```python
from build123d import *

# Parameters (mm, degrees)
CYLINDER005_R     = 2.2
CYLINDER005_DEPTH = 32
ARRAY004_X_COUNT  = 2
ARRAY004_X_PITCH  = 40
ARRAY004_Y_COUNT  = 2
ARRAY004_Y_PITCH  = 90
BOX005_W          = 62
BOX005_H          = 108
BOX005_DEPTH      = 32


with BuildPart() as psu_mockup_hole_array:
    # Cylinder005 → Cylinder005 (new body)
    with BuildSketch(Plane.XY):
        Circle(CYLINDER005_R)
    extrude(amount=CYLINDER005_DEPTH)

    # Array004 X: psu mockup hole array ×2


with BuildPart() as psu_mockup_hole_array_1:
    add(psu_mockup_hole_array.part)
    with Locations(*[(i * ARRAY004_X_PITCH, 0, 0) for i in range(1, ARRAY004_X_COUNT)]):
        add(psu_mockup_hole_array.part)

    # Array004 Y: psu mockup hole array ×2


with BuildPart() as psu_mockup_hole_array_2:
    add(psu_mockup_hole_array_1.part)
    with Locations(*[(0, i * ARRAY004_Y_PITCH, 0) for i in range(1, ARRAY004_Y_COUNT)]):
        add(psu_mockup_hole_array_1.part)


with BuildPart() as psu_mockup_hole_array_3:
    # Array004 placement: moved
    add(psu_mockup_hole_array_2.part.moved(Location((11, 9, 0))))


with BuildPart() as psu_mockup_with_holes:
    # Box005 → Box005 (new body)
    with BuildSketch(Plane.XY):
        with Locations((31, 54)):
            Rectangle(BOX005_W, BOX005_H)
    extrude(amount=BOX005_DEPTH)

    # Cut003: cut psu mockup hole array
    add(psu_mockup_hole_array_3.part, mode=Mode.SUBTRACT)


with BuildPart() as psu_mockup_with_holes_1:
    # Cut003 placement: moved
    add(psu_mockup_with_holes.part.moved(Location((-31, 40, 10))))


solid = psu_mockup_with_holes_1.part
```
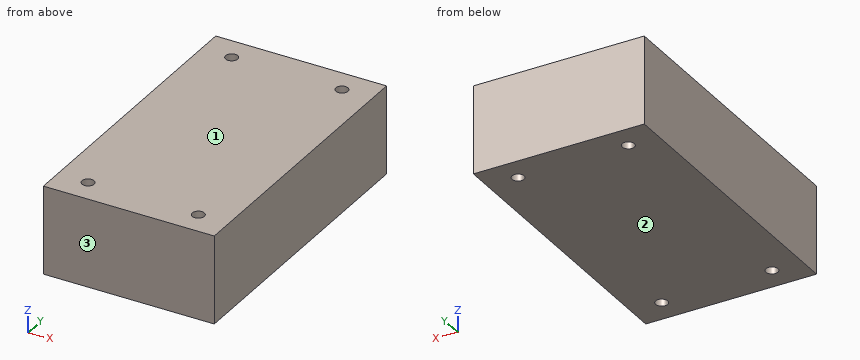
Here's how the part is built. I have some questions about the finished solid (model axes, mm). Face numbers are marked on the shaded views. Round coordinates to 2 decimals unless told otherwise and drop trailing zeros. Order: outer loops, then holes, each group sorted by start corner. A loop starts at its lowest first (then second) coordinate and runs counter-clockwise, first axis right, second up. Notation, with made-up numbers: M 35.5,54.5 L 66.5,54.5 A9 cw 66.5,68.5 Z; hole C -15.75,82.25 d9. An arc over 180 degrees is marked long. One line per question, with ' | ' between items.
1) I want a section at A-A, the plane x = 20. Write out the boundary of the cut face in (y, z).
Working result:
outline: M 40,10 L 46.8,10 L 46.8,42 L 40,42 Z; M 51.2,10 L 136.8,10 L 136.8,42 L 51.2,42 Z; M 141.2,10 L 148,10 L 148,42 L 141.2,42 Z
2) I want a section at B-B, the plane y = 139. Write out the boundary of the cut face in (x, z).
Working result:
outline: M -31,10 L -22.2,10 L -22.2,42 L -31,42 Z; M -17.8,10 L 17.8,10 L 17.8,42 L -17.8,42 Z; M 22.2,10 L 31,10 L 31,42 L 22.2,42 Z
3) If we mould it in two halves opening along Z, with no side actions, what happens to the marked faces 1, 2 and 3? For each: +Z half, -Z half, draft (parallel to the pull), parting line (faces both ways), or undercut.
Working result:
face 1: +Z half | face 2: -Z half | face 3: draft
4) For pin 1 Ø2.5 at (x, y) = (-20, 139) entering from -Z, with a flat end and sliding along its axis, tell me the tip position at first contact or that it passes through.
Working result:
pin 1: through
5) I need wall thicknesses on line 1 along X through (y, z) = (139, 34); line 2 along Y through (x, z) = (-20, 24). Which ranges of each line are inside material? Lowest first, please.
Working result:
line 1: -31 to -22.2, -17.8 to 17.8, 22.2 to 31 | line 2: 40 to 46.8, 51.2 to 136.8, 141.2 to 148
